The figure shows three views and two pictorial views of one solid part (mm, origin at its lowest corner). Answer the questions. A direction names the side the tool comes from. Coordinates: 2 decimals unless noted, no trailing zeros. Loops run counter-clockwise (first coordinate to the right, second up) from the corner with the lowest first, then second, coordinate; pieces in that order, holes last. Notation, with made-up numbers: (64, 45.5) - (119, 45.5) arc R21 ccw to (119, 63.5) - close; hole circle Ø2 at (40.25, -19). An arc over 180 degrees is marked (long way). Write each question's results on one line, items separated by ' | '. Start each with the question number.
Item 1: A tool of negligible diameter and unlimited length cuts with its end or side. For the marked faces 1, 2 and 3, from which of +Z, -Z, +X, -X, +Y, -Y can it reach the whole face along a straight path? Write none if from no direction.
Item 2: Consider probe 1 along Y at (x, z) = (3.95, 0.3); probe 2 along Y at (x, z) = (3.15, 2.7); probe 3 along X at (y, z) = (0.5, 2.3) (1 decimal). Determine where each line is inside the solid, lowest interval first. Write a range as [from, to].
Item 3: Section A-A, the plane z = 2.9 is taken. Write down the section's boundary in (x, y), plus the area to 3 significant figures.
Item 4: For a pull along Z with two mould halves and no side action, classify the marked faces 4, 5 and 6 as +Z half, -Z half, draft (parallel to the pull), parting line (faces both ways), or undercut.
Item 5: Each of these flat-tipped pins is pushed along its axis until it touches: pin 1 Ø0.6 at (x, z) = (3, 2.5) entering from -Y; pin 2 Ø2 at (y, z) = (2.5, 3.5) entering from +X. Where does it stop, or does it pass through?
Item 6: Section D-D, the plane z = 1.65 is taken. Write down the section's boundary in (x, y), plus the area to 3 significant figures.
Item 7: Section B-B, the plane y = 2 is taken. Write down the section's boundary in (x, z).
Item 8: Section C-C, the plane x = 1.2 is taken. Write down the section's boundary in (y, z).
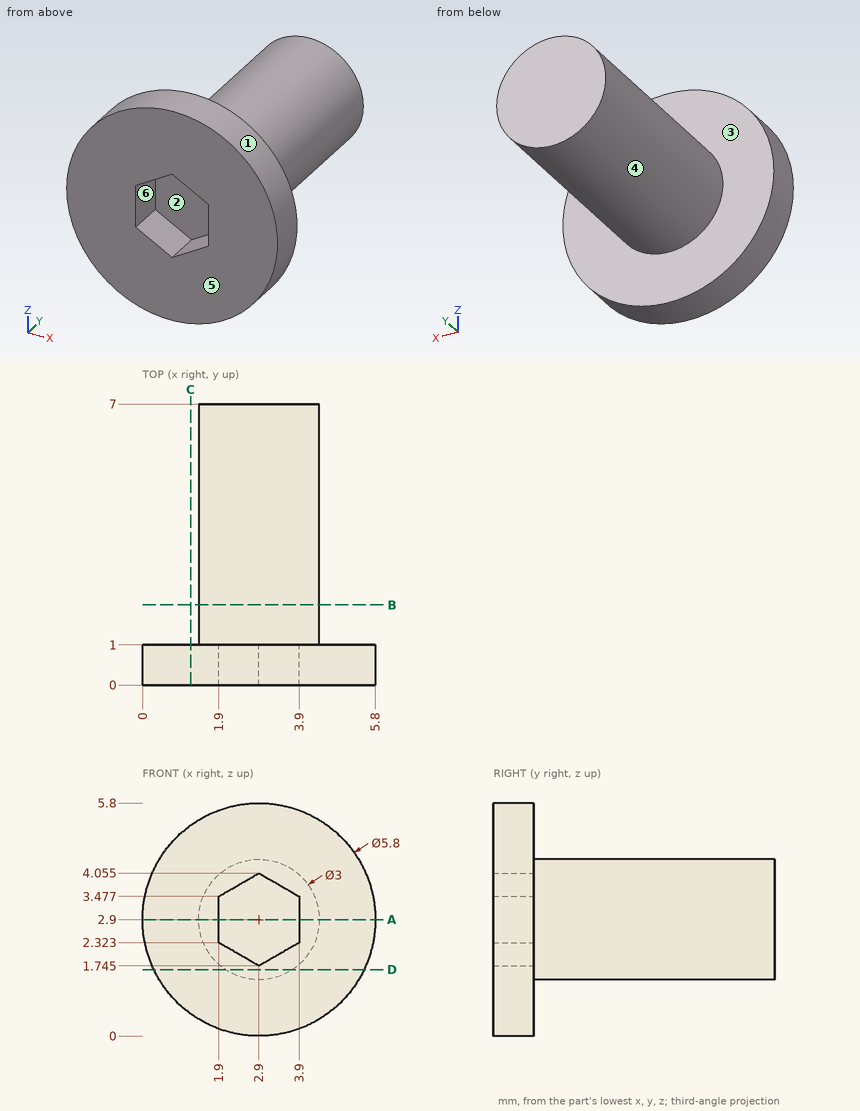
Answer key:
1) face 1: +Y, -Y | face 2: -Y | face 3: +Y
2) probe 1: y = [0, 1] | probe 2: y = [1, 7] | probe 3: x = [0.1, 1.9], [3.9, 5.7]
3) outline: (0, 0) - (1.9, 0) - (1.9, 1) - (3.9, 1) - (3.9, 0) - (5.8, 0) - (5.8, 1) - (4.4, 1) - (4.4, 7) - (1.4, 7) - (1.4, 1) - (0, 1) - close | area: 21.8 mm^2
4) face 4: parting line | face 5: draft | face 6: undercut
5) pin 1: stops at y = 1 | pin 2: stops at x = 4.4
6) outline: (0.28, 0) - (5.52, 0) - (5.52, 1) - (3.73, 1) - (3.73, 7) - (2.07, 7) - (2.07, 1) - (0.28, 1) - close | area: 15.2 mm^2
7) outline: circle Ø3 at (2.9, 2.9)
8) outline: (0, 0.55) - (1, 0.55) - (1, 5.25) - (0, 5.25) - close
